```python
from build123d import *

# Parameters (mm, degrees)
EXTRUDE_1_DEPTH      = 70
SKETCH_3_W           = 10
SKETCH_3_H           = 30
CUT_EXTRUDE_2_DEPTH  = 92.104335791
CUT_EXTRUDE_3_DEPTH  = 87.02325267
SKETCH_5_W           = 10
SKETCH_5_H           = 25
CUT_EXTRUDE_4_DEPTH  = 83.607505712
SKETCH_8_W           = 32
SKETCH_8_H           = 25
CUT_EXTRUDE_5_DEPTH  = 27
CUT_EXTRUDE_6_DEPTH  = 81.802227692
SKETCH_10_R          = 6.3
CUT_EXTRUDE_7_DEPTH  = 6
SKETCH_11_R          = 2.5
CUT_EXTRUDE_8_DEPTH  = 63.801273872
SKETCH_12_R          = 2
CUT_EXTRUDE_9_DEPTH  = 87.02325267
CUT_EXTRUDE_10_REACH = 88.023
SKETCH_13_R          = 2
CUT_EXTRUDE_11_DEPTH = 10
SKETCH_15_W          = 12
SKETCH_15_H          = 32
EXTRUDE_2_DEPTH      = 20
CUT_EXTRUDE_12_DEPTH = 63.801273872
CUT_EXTRUDE_13_DEPTH = 32
SKETCH_18_W          = 20
SKETCH_18_H          = 32
CUT_EXTRUDE_14_DEPTH = 85.409715081
EXTRUDE_3_DEPTH      = 28
SKETCH_21_W          = 10
SKETCH_21_H          = 5
CUT_EXTRUDE_15_DEPTH = 85.551759296
CHAMFER_1_SIZE       = 1
CHAMFER_2_SIZE       = 1
SKETCH_22_R          = 2
CUT_EXTRUDE_16_DEPTH = 20


with BuildPart() as part:
    # 草图1 → 拉伸1 (new body)
    with BuildSketch(Plane.XY):
        Polygon((0, 0), (50, 0), (50, 30), (30, 30), align=None)
    extrude(amount=EXTRUDE_1_DEPTH)

    # 草图3 → 切除-拉伸2 (cut, through all)
    with BuildSketch(Plane.XY.offset(70)):
        with Locations((45, 15)):
            Rectangle(SKETCH_3_W, SKETCH_3_H)
    extrude(amount=-CUT_EXTRUDE_2_DEPTH, mode=Mode.SUBTRACT)

    # 草图4 → 切除-拉伸3 (cut, through all)
    with BuildSketch(Plane.XY.offset(70)):
        Polygon((0, 0), (8, 8), (8, 0), align=None)
    extrude(amount=-CUT_EXTRUDE_3_DEPTH, mode=Mode.SUBTRACT)

    # 草图5 → 切除-拉伸4 (cut, through all)
    with BuildSketch(Plane(origin=(40, 0, 0), x_dir=(0, 0, -1), z_dir=(1, 0, 0))):
        with Locations((-65, 17.5)):
            Rectangle(SKETCH_5_W, SKETCH_5_H)
        with Locations((-45, 17.5)):
            Rectangle(SKETCH_5_W, SKETCH_5_H)
    extrude(amount=-CUT_EXTRUDE_4_DEPTH, mode=Mode.SUBTRACT)

    # 草图8 → 切除-拉伸5 (cut)
    with BuildSketch(Plane.ZY.offset(-8)):
        with Locations((16, 17.5)):
            Rectangle(SKETCH_8_W, SKETCH_8_H)
    extrude(amount=-CUT_EXTRUDE_5_DEPTH, mode=Mode.SUBTRACT)

    # 草图9 → 切除-拉伸6 (cut, through all)
    with BuildSketch(Plane.ZY.offset(-35)):
        Polygon((0, 30), (32, 30), (0, 5), align=None)
    extrude(amount=-CUT_EXTRUDE_6_DEPTH, mode=Mode.SUBTRACT)

    # 草图10 → 切除-拉伸7 (cut)
    with BuildSketch(Plane(origin=(0, 0, 32), x_dir=(-1, 0, 0), z_dir=(0, 0, -1))):
        with Locations((-32, 23)):
            Circle(SKETCH_10_R)
    extrude(amount=-CUT_EXTRUDE_7_DEPTH, mode=Mode.SUBTRACT)

    # 草图11 → 切除-拉伸8 (cut, through all)
    with BuildSketch(Plane(origin=(0, 0, 38), x_dir=(-1, 0, 0), z_dir=(0, 0, -1))):
        with Locations((-32, 23)):
            Circle(SKETCH_11_R)
    extrude(amount=-CUT_EXTRUDE_8_DEPTH, mode=Mode.SUBTRACT)

    # 草图12 → 切除-拉伸9 (cut, through all)
    with BuildSketch(Plane.XZ):
        with Locations(Location((14, 10, 0), (0, 0, 270))):
            Circle(SKETCH_12_R)
    extrude(amount=-CUT_EXTRUDE_9_DEPTH, mode=Mode.SUBTRACT)

    # 草图13 → 切除-拉伸10 (cut, up to next)
    with BuildSketch(Plane.XZ, mode=Mode.PRIVATE) as cut_extrude_10_sk1:
        with Locations(Location((34, 65, 0), (0, 0, 270))):
            Circle(SKETCH_13_R)
    cut_extrude_10_tool1 = extrude(cut_extrude_10_sk1.sketch, amount=-CUT_EXTRUDE_10_REACH, mode=Mode.PRIVATE) & part.part
    add(cut_extrude_10_tool1.solids().sort_by_distance((34, 0, 65))[0], mode=Mode.SUBTRACT)

    # 草图14 → 切除-拉伸11 (cut)
    with BuildSketch(Plane.ZY.offset(-35)):
        Polygon((32, 30), (32, 5), (0, 5), align=None)
    extrude(amount=-CUT_EXTRUDE_11_DEPTH, mode=Mode.SUBTRACT)

    # 草图15 → 拉伸2 (add)
    with BuildSketch(Plane(origin=(0, 5, 0), x_dir=(-1, 0, 0), z_dir=(0, 1, 0))):
        with Locations((-14, 16)):
            Rectangle(SKETCH_15_W, SKETCH_15_H)
    extrude(amount=EXTRUDE_2_DEPTH)

    # 草图16 → 切除-拉伸12 (cut, through all)
    with BuildSketch(Plane.XY.offset(32)):
        Polygon((20, 25), (20, 20), (8, 8), (8, 25), align=None)
    extrude(amount=-CUT_EXTRUDE_12_DEPTH, mode=Mode.SUBTRACT)

    # 草图17 → 切除-拉伸13 (cut)
    with BuildSketch(Plane(origin=(0, 0, 0), x_dir=(-1, 0, 0), z_dir=(0, 0, -1))):
        Polygon((-20, 20), (-20, 17), (-17, 17), align=None)
    extrude(amount=-CUT_EXTRUDE_13_DEPTH, mode=Mode.SUBTRACT)

    # 草图18 → 切除-拉伸14 (cut, through all)
    with BuildSketch(Plane(origin=(0, 5, 0), x_dir=(-1, 0, 0), z_dir=(0, 1, 0))):
        with Locations((-30, 16)):
            Rectangle(SKETCH_18_W, SKETCH_18_H)
    extrude(amount=-CUT_EXTRUDE_14_DEPTH, mode=Mode.SUBTRACT)

    # 草图20 → 拉伸3 (add)
    with BuildSketch(Plane.XY.offset(60)):
        Polygon((30, 30), (35, 35), (40, 35), (40, 30), align=None)
    extrude(amount=-EXTRUDE_3_DEPTH)

    # 草图21 → 切除-拉伸15 (cut, through all)
    with BuildSketch(Plane(origin=(40, 0, 0), x_dir=(0, 0, -1), z_dir=(1, 0, 0))):
        with Locations((-45, 32.5)):
            Rectangle(SKETCH_21_W, SKETCH_21_H)
    extrude(amount=-CUT_EXTRUDE_15_DEPTH, mode=Mode.SUBTRACT)

    # 倒角1
    chamfer_1_edges = [part.edges().sort_by_distance(p)[0] for p in [
        (37.5, 35, 60),
        (37.5, 35, 32),
        (37.5, 35, 40),
        (37.5, 35, 50),
    ]]
    chamfer(chamfer_1_edges, length=CHAMFER_1_SIZE)

    # 倒角2
    chamfer_2_edges = [part.edges().sort_by_distance(p)[0] for p in [
        (40, 35, 36),
        (40, 35, 55),
    ]]
    chamfer(chamfer_2_edges, length=CHAMFER_2_SIZE)

    # 草图22 → 切除-拉伸16 (cut)
    with BuildSketch(Plane.XZ.offset(-5)):
        with Locations(Location((14, 10, 0), (0, 0, 270))):
            Circle(SKETCH_22_R)
    extrude(amount=-CUT_EXTRUDE_16_DEPTH, mode=Mode.SUBTRACT)


solid = part.part
```
Can you work these out from the model? Positions are in its coordinate system, mm. A direction names the side the tool comes from. Coordinates: 2 decimals unless noted, no trailing zeros. Write each loop counter-clockwise with the first axis right and the second up, starting at its lowest first coordinate (ties: lowest second). Pieces come first, ordered by that corner, then holes. Notation, with made-up numbers: M -10,-10 L 19,-10 A36 ccw 19,29 Z; hole C 35.25,65 d10. An arc over 180 degrees is marked long. Write item = value, one per line. Start each with the question number.
Q1. If I drill on L1, parallel to Z at x = 14, y = 9; L2, parallel to Z at x = 21.5, y = 12; L3, parallel to Y at x = 32, z = 39.05, over which ranges is the centre line in solid material (lowest first)? Write a range as [from, to].
Q2. If we section it at A-A, the plane y = 32: Write out the boundary of the cut face in (x, z), then the cut area to 3 significant figures.
Q3. Thinking about a two-plate mould opening in Y: for faces 1 (the face through (32.33, 25.48, 38.99)), 2 (the face through (20, 0, 42)), 3 (the face through (15, 15, 25)), which applies, released by +Y, released by -Y, zero draft, split by the parting line, or undercut?
Q4. On a 3-axis mill with a long thin cutter (end or side, diameter ignored), from which of +Z, -Z, +X, -X, +Y, -Y can I reach the whole of each face in a straight line? I mean faces 4 (the face through (20, 8, 16)), 5 (the face through (32, 20, 38)), 6 (the face through (28, 16, 60)), 7 (the face through (28, 16, 50)). Say none if no direction works.
Q5. If we section it at D-D, the plane z = 10: Write out the boundary of the cut face in (x, y), then the cut area to 4 significant figures.
Q6. If we section it at C-C, the plane y = 23: Write out the boundary of the cut face in (x, z), then the cut area to 3 significant figures.
Q7. If we section it at B-B, the plane x = 14: Write out the boundary of the cut face in (y, z), then the cut area to 3 significant figures.
Q8. I'm going to push flat-ended pins straight in: pin 1 (18.5 mm diameter, centred on x = 30, y = 25.5, fed in from -Z); pin 2 (4 mm diameter, centred on x = 34.5, y = 23.5, fed in from -Z); pin 3 (3 mm diameter, centred on x = 21.5, z = 47.5, fed in from +Y). Where does each tip first touch, or does it pass through?
Check sheet entries:
q1.L1 = [0, 8], [12, 40], [50, 60]
q1.L2 = [32, 40], [50, 60]
q1.L3 = [0, 20.5], [25.5, 32]
q2.outline = M 32,32 L 40,32 L 40,40 L 32,40 Z; M 32,50 L 40,50 L 40,60 L 32,60 Z
q2.area = 144 mm²
q3.face_1 = undercut
q3.face_2 = released by -Y
q3.face_3 = released by +Y
q4.face_4 = -Z, +X, +Y, -Y
q4.face_5 = -Z
q4.face_6 = +Z, +X, -X, +Y
q4.face_7 = +X, -X, +Y
q5.outline = M 8,0 L 12,0 L 12,12 L 8,8 Z; M 16,0 L 20,0 L 20,17 L 17,17 L 16,16 Z
q5.area = 107.5 mm²
q6.outline = M 23,32 L 25.7,32 L 25.7,38 L 29.5,38 L 29.5,40 L 23,40 Z; M 23,50 L 29.5,50 L 29.5,60 L 23,60 Z; M 34.5,38 L 38.3,38 L 38.3,32 L 40,32 L 40,40 L 34.5,40 Z; M 34.5,50 L 40,50 L 40,60 L 34.5,60 Z
q6.area = 170 mm²
q7.outline = M 0,0 L 14,0 L 14,8 L 0,8 Z; M 0,12 L 14,12 L 14,40 L 5,40 L 5,50 L 14,50 L 14,60 L 5,60 L 5,70 L 0,70 Z
q7.area = 744 mm²
q8.pin_1 = 32
q8.pin_2 = 38
q8.pin_3 = 5
